Input: part model. Units: mm. Frame: model coordinates. A direction names the side the tool comes from. Give positions to 0.01 mm unless a question says otherwise; leave off trailing zeros. Order: outer loops, then holes, each group sorted by start corner. A loop starts at its lowest first (then second) coordinate and runs counter-clockwise, first axis right, second up. Notation, with made-up numbers: (36.25, -13) - (87.25, -13) arc R25 ccw to (87.25, 26) - close; hole circle Ø2 at (55.5, 87). An arc over 180 degrees is marked (long way). Use a Markdown table: item, result.
from build123d import *

# Parameters (mm, degrees)
BOSS_EXTRUDE1_DEPTH = 5
SKETCH2_W           = 5
SKETCH2_H           = 20
BOSS_EXTRUDE2_DEPTH = 8
SKETCH3_R           = 2.1
CUT_EXTRUDE1_DEPTH  = 8
FILLET2_R           = 2
SKETCH4_W           = 5
SKETCH4_H           = 5
CUT_EXTRUDE2_DEPTH  = 3
FILLET3_R           = 3


with BuildPart() as part:
    # Sketch1 → Boss-Extrude1 (new body)
    with BuildSketch(Plane(origin=(0, 0, 0), x_dir=(1, 0, 0), z_dir=(0, 1, 0))):
        with BuildLine():
            Line((-5, 0), (-5, 13.835803565))
            ThreePointArc((-5, 13.835803565), (0, 18.835803565), (5, 13.835803565))
            Line((5, 13.835803565), (5, 0))
            Line((5, 0), (5, -45))
            Line((5, -45), (-5, -45))
            Line((-5, -45), (-5, 0))
        make_face()
        with BuildLine():
            Line((-2.1, -8), (-2.1, 13.835803565))
            ThreePointArc((-2.1, 13.835803565), (0, 15.935803565), (2.1, 13.835803565))
            Line((2.1, 13.835803565), (2.1, -8))
            ThreePointArc((2.1, -8), (0, -10.1), (-2.1, -8))
        make_face(mode=Mode.SUBTRACT)
    extrude(amount=BOSS_EXTRUDE1_DEPTH)

    # Sketch2 → Boss-Extrude2 (add)
    with BuildSketch(Plane.XY.offset(45)):
        with Locations((2.5, 2.5)):
            Rectangle(SKETCH2_W, SKETCH2_H)
    extrude(amount=BOSS_EXTRUDE2_DEPTH)

    # Sketch3 → Cut-Extrude1 (cut)
    with BuildSketch(Plane(origin=(5, 0, 0), x_dir=(0, 0, -1), z_dir=(1, 0, 0))):
        with Locations((-49, 8.5)):
            Circle(SKETCH3_R)
        with Locations((-49, -3.5)):
            Circle(SKETCH3_R)
    extrude(amount=-CUT_EXTRUDE1_DEPTH, mode=Mode.SUBTRACT)

    # Fillet2
    fillet2_edges = [part.edges().sort_by_distance(p)[0] for p in [
        (2.5, 12.5, 45),
        (2.5, -7.5, 45),
        (2.5, 12.5, 53),
        (2.5, -7.5, 53),
    ]]
    fillet(fillet2_edges, radius=FILLET2_R)

    # Sketch4 → Cut-Extrude2 (cut)
    with BuildSketch(Plane.XY.offset(45)):
        with Locations((-2.5, 2.5)):
            Rectangle(SKETCH4_W, SKETCH4_H)
    extrude(amount=-CUT_EXTRUDE2_DEPTH, mode=Mode.SUBTRACT)

    # Fillet3
    fillet3_edges = [part.edges().sort_by_distance(p)[0] for p in [
        (2.5, 0, 45),
        (2.5, 5, 45),
        (-5, 2.5, 42),
    ]]
    fillet(fillet3_edges, radius=FILLET3_R)


solid = part.part
1. Mould query, pull axis Y, two halves, no side actions, for faces 1 (the face through (2.54, -4.3, 47.06)), 2 (the face through (0, 5, 11)), 3 (the face through (0, 2, 49)), 4 (the face through (2, -7.5, 49)). Classes: pulls with the +Y half, pulls with the -Y half, needs draft (parallel to the pull), parting line crosses it, or undercut.
Response:
| item | result |
|---|---|
| face 1 | undercut |
| face 2 | pulls with the +Y half |
| face 3 | needs draft |
| face 4 | pulls with the -Y half |
2. Set-up query: faces 5 (the face through (-0.046, 2.465, -15.935)), 6 (the face through (0, 0, 11)), 7 (the face through (2.54, 11.93, 45.6)). Return all of +Z, -Z, +X, -X, +Y, -Y with unobstructed straight access to the full face (end or side cutting, diameter ignored); none if empty.
Response:
| item | result |
|---|---|
| face 5 | +Y, -Y |
| face 6 | -Z, +X, -X, -Y |
| face 7 | -Z, +X, -X, +Y |
3. Section query B-B (z = 49). Return loops of the section in (x, y).
Response:
| item | result |
|---|---|
| outline | (0, -7.5) - (5, -7.5) - (5, -5.6) - (0, -5.6) - close; (0, -1.4) - (5, -1.4) - (5, 6.4) - (0, 6.4) - close; (0, 10.6) - (5, 10.6) - (5, 12.5) - (0, 12.5) - close |
4. Section query A-A (z = -11). Return loops of the section in (x, y), then the cut area to 3 significant figures.
Response:
| item | result |
|---|---|
| outline | (-5, 0) - (-2.1, 0) - (-2.1, 5) - (-5, 5) - close; (2.1, 0) - (5, 0) - (5, 5) - (2.1, 5) - close |
| area | 29.0 mm^2 |
5. Pin query (flat end, axial travel): pin 1 (3 mm diameter, centred on x = -1.5, z = 29.5, fed in from +Y); pin 2 (2.5 mm diameter, centred on y = 8.5, z = 49, fed in from -X) (3 decimals); pin 3 (5.5 mm diameter, centred on y = 6, z = 48, fed in from -X); pin 4 (6 mm diameter, centred on x = -2.5, z = 41, fed in from -Y). Return the tip coordinate at first contact, or that it passes through.
Response:
| item | result |
|---|---|
| pin 1 | stops at y = 5 |
| pin 2 | passes through |
| pin 3 | stops at x = 0 |
| pin 4 | stops at y = -0.07 |
6. Section query C-C (y = 3). Return loops of the section in (x, z), then the cut area to 3 significant figures.
Response:
| item | result |
|---|---|
| outline | (-5, -13.84) arc R5 ccw to (5, -13.84) - (5, 53) - (0, 53) - (0, 42) - (-2, 42) arc R3 ccw to (-5, 39) - close; hole (-2.1, -13.84) arc R2.1 ccw to (2.1, -13.84) - (2.1, 8) arc R2.1 ccw to (-2.1, 8) - close |
| area | 545 mm^2 |
7. Material intervals for line 1 along Y through (x, z) = (2.8, 49); line 2 along Y through (x, z) = (0.5, 50); line 3 along X through (y, z) = (3.25, 4), sorted ascending.
Response:
| item | result |
|---|---|
| line 1 | y = -7.5 to -5.6, -1.4 to 6.4, 10.6 to 12.5 |
| line 2 | y = -7.5 to -5.35, -1.65 to 6.65, 10.35 to 12.5 |
| line 3 | x = -5 to -2.1, 2.1 to 5 |
8. Section query D-D (y = -4.75). Return loops of the section in (x, z).
Response:
| item | result |
|---|---|
| outline | (0, 45) - (5, 45) - (5, 47.31) - (0, 47.31) - close; (0, 50.69) - (5, 50.69) - (5, 53) - (0, 53) - close |
